Geometry check sheet. Reference: the model listing, model coordinates, mm. Face numbers are marked on the shaded views. Give positions to 0.01 mm unless a question says otherwise; leave off trailing zeros. Order: outer loops, then holes, each group sorted by start corner. A loop starts at its lowest first (then second) coordinate and runs counter-clockwise, first axis right, second up. Notation, with made-up numbers: (16, 47) - (70, 47) arc R23 ccw to (70, 73) - close; hole circle Ø2 at (-10.75, 27.5). An arc over 180 degrees is marked (long way). Put each result on its own line as item: value. Start each with the question number.
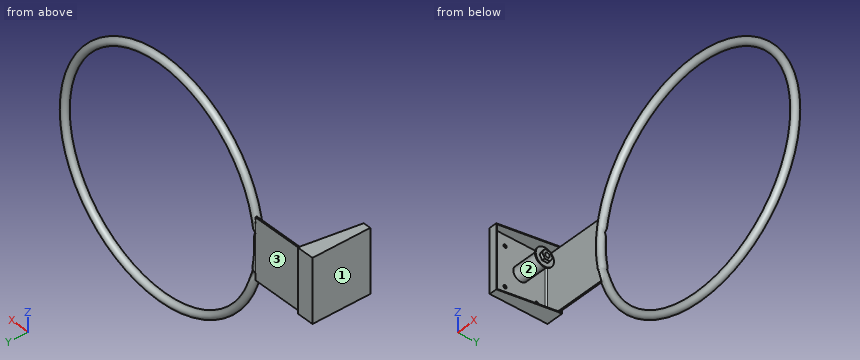
Autodesk Inventor part; units mm, degrees
ref_plane "YZ Plane" through (0, 0, 0) normal (1, 0, 0) x (0, 1, 0)
ref_plane "XZ Plane" through (0, 0, 0) normal (0, 1, 0) x (-1, 0, 0)
ref_plane "XY Plane" through (0, 0, 0) normal (0, 0, 1) x (1, 0, 0)
sketch "Sketch1" plane through (0, 0, 0) normal (0, 0, 1) x (1, 0, 0)
  circle A0 centre (0, 0) radius 7.9375
  line L0 (236.5375, 47.7842) -> (236.5375, -114.9552)
  dimension "d0" = 228.6
  dimension "d1" = 15.875
revolve "Revolution1" add sketch "Sketch1" angle 360 about axis through (236.5375, 47.7842, 0) along (0, -1, 0)
sketch "Sketch2" plane through (0, 0, 0) normal (0, 0, 1) x (1, 0, 0)
  line L0 (0, 4.7625) -> (-134.9375, 4.7625)
  line L1 (-138.1125, 1.5875) -> (-138.1125, -106.3625)
  line L2 (-138.1125, -106.3625) -> (-141.2875, -106.3625)
  line L3 (-141.2875, -106.3625) -> (-141.2875, 1.5875)
  line L4 (-134.9375, 7.9375) -> (0, 7.9375)
  line L5 (0, 7.9375) -> (0, 4.7625)
  arc A0 (-134.9375, 4.7625) -> (-138.1125, 1.5875) centre (-134.9375, 1.5875) ccw
  arc A1 (-134.9375, 7.9375) -> (-141.2875, 1.5875) centre (-134.9375, 1.5875) ccw
  point P0 (0, 0)
  point P1 (-138.1125, 4.7625)
  dimension "d5" = 0
  dimension "d6" = 7.9375
  dimension "d7" = 3.175
  dimension "d8" = 3.175
  dimension "d9" = 6.35
  dimension "d27" = 114.3
  dimension "d28" = 141.2875
extrude "Extrusion1" add sketch "Sketch2" along normal mid plane 125.4125
sketch "Sketch3" plane through (-141.2875, -106.3625, 62.7062) normal (-1, 0, 0) x (0, 0, 1)
  line L0 (0, 0) -> (0, 107.95)
  line L1 (0, 107.95) -> (-125.4125, 107.95)
  line L2 (-125.4125, 107.95) -> (-125.4125, 0)
  line L3 (0, 0) -> (-125.4125, 0)
  line L4 (0, 114.3) -> (-125.4125, 114.3)
  line L5 (-125.4125, 107.95) -> (-125.4125, 114.3)
  line L6 (0, 114.3) -> (0, 107.95)
  arc A0 (-103.9113, 100.9746) -> (-110.4012, 84.7629) centre (-107.1562, 92.8687) ccw
  arc A1 (-102.47, 81.5879) -> (-95.9802, 97.7996) centre (-99.2251, 89.6937) ccw
  arc A2 (-29.4323, 97.7996) -> (-22.9425, 81.5879) centre (-26.1874, 89.6937) ccw
  arc A3 (-15.0113, 84.7629) -> (-21.5012, 100.9746) centre (-18.2562, 92.8687) ccw
  arc A4 (-110.4012, 31.1246) -> (-103.9113, 14.9129) centre (-107.1562, 23.0187) ccw
  arc A5 (-95.9802, 18.0879) -> (-102.47, 34.2996) centre (-99.2251, 26.1937) ccw
  arc A6 (-22.9425, 34.2996) -> (-29.4323, 18.0879) centre (-26.1874, 26.1937) ccw
  arc A7 (-21.5012, 14.9129) -> (-15.0113, 31.1246) centre (-18.2562, 23.0187) ccw
  line L7 (-110.4012, 84.7629) -> (-102.47, 81.5879)
  line L8 (-103.9113, 100.9746) -> (-95.9802, 97.7996)
  line L9 (-21.5012, 100.9746) -> (-29.4323, 97.7996)
  line L10 (-15.0113, 84.7629) -> (-22.9425, 81.5879)
  line L11 (-22.9425, 34.2996) -> (-15.0113, 31.1246)
  line L12 (-21.5012, 14.9129) -> (-29.4323, 18.0879)
  line L13 (-103.9113, 14.9129) -> (-95.9802, 18.0879)
  line L14 (-102.47, 34.2996) -> (-110.4012, 31.1246)
  line L15 (-107.1562, 23.0187) -> (-107.1562, 92.8687)
  line L16 (-99.2251, 26.1937) -> (-99.2251, 89.6937)
  line L17 (-26.1874, 26.1937) -> (-26.1874, 89.6937)
  line L18 (-18.2562, 23.0187) -> (-18.2562, 92.8687)
  line L19 (-99.2251, 89.6937) -> (-26.1874, 89.6937)
  line L20 (-107.1562, 92.8687) -> (-18.2562, 92.8687)
  line L21 (-99.2251, 26.1937) -> (-26.1874, 26.1937)
  line L22 (-107.1562, 23.0187) -> (-18.2562, 23.0187)
  dimension "d29" = 106.3625
  dimension "d30" = 55.5752
  dimension "d31" = 87.3125
  dimension "d32" = 46.0375
  dimension "d33" = 17.4625
  dimension "d34" = 9.525
  dimension "d35" = 12.7
  dimension "d36" = 9.525
  dimension "d37" = 33.3375
  dimension "d38" = 79.375
  dimension "d39" = 34.9186
hole "Hole1" at (-138.1125, -15.0812, 40.4812) direction (-1, 0, 0) diameter 6.731 end through all
pattern_linear "Rectangular Pattern1" count 2 spacing 80.9625 along (0, 0, -1) count 2 spacing 66.675 along (0, -1, 0) of "Hole1"
hole "Hole2" at (-141.2875, -49.2125, 0.7937) direction (1, 0, 0) diameter 12.7 depth 25.4 tip angle 118
sketch "Sketch4" plane through (-141.2875, -106.3625, 62.7062) normal (-1, 0, 0) x (0, 0, 1)
  line L0 (0, 0) -> (0, 107.95)
  line L1 (-125.4125, 107.95) -> (-125.4125, 0)
  line L2 (0, 0) -> (-125.4125, 0)
  line L3 (-128.5875, -3.175) -> (3.175, -3.175)
  line L4 (3.175, -3.175) -> (3.175, 117.475)
  line L5 (3.175, 117.475) -> (-128.5875, 117.475)
  line L6 (-128.5875, 117.475) -> (-128.5875, -3.175)
  line L7 (0, 114.3) -> (-125.4125, 114.3)
  line L8 (-127, 115.8875) -> (1.5875, 115.8875)
  line L9 (1.5875, 115.8875) -> (1.5875, -1.5875)
  line L10 (1.5875, -1.5875) -> (-127, -1.5875)
  line L11 (-127, -1.5875) -> (-127, 115.8875)
  point P0 (-62.7062, 106.3625)
  dimension "d49" = 3.175
  dimension "d50" = 3.175
  dimension "d51" = 3.175
  dimension "d52" = 3.175
  dimension "d53" = 1.5875
extrude "Extrusion2" add sketch "Sketch4" along normal blind 1.5875 contours L6 L5 L4 L3 | L8 L9 L10 L11
extrude "Extrusion3" add sketch "Sketch4" against normal blind 33.3375
sketch "Sketch8" plane through (-142.875, -109.5375, 65.8813) normal (0, 0, 1) x (1, 0, 0)
  line L0 (0, 120.65) -> (0, 0)
  line L1 (34.925, 0) -> (0, 0)
  line L2 (34.925, 0) -> (34.925, 120.65)
  line L3 (34.925, 120.65) -> (0, 120.65)
  line L4 (34.925, 114.3) -> (15.875, 0)
  line L5 (34.925, 0) -> (34.925, 114.3)
  line L6 (15.875, 0) -> (34.925, 0)
  point P0 (142.875, 109.5375)
  dimension "d67" = 6.35
  dimension "d68" = 15.875
extrude "Extrusion7" cut sketch "Sketch8" against normal through all contours L4 L2 L1
sketch "Sketch5" plane through (-141.2875, -49.2125, 0.7937) normal (1, 0, 0) x (0, 0, -1)
  circle A0 centre (0, 0) radius 6.35
  circle A1 centre (0, 0) radius 4.7625
  point P0 (0.7937, 49.2125)
  dimension "d58" = 9.525
extrude "Extrusion4" add sketch "Sketch5" along normal blind 60.325 contours A1
sketch "Sketch6" plane through (-80.9625, -49.2125, 0.7937) normal (1, 0, 0) x (0, 0, -1)
  circle A0 centre (0, 0) radius 4.7625
  circle A1 centre (0, 0) radius 19.05
  point P0 (0.7937, 49.2125)
  dimension "d61" = 38.1
extrude "Extrusion5" add sketch "Sketch6" along normal blind 1.905
sketch "Sketch7" plane through (-79.0575, -49.2125, 0.7937) normal (1, 0, 0) x (0, 0, -1)
  circle A0 centre (0, 0) radius 4.7625
  circle A1 centre (0, 0) radius 19.05
  line L0 (0, 10.9985) -> (9.525, 5.4993)
  line L1 (9.525, 5.4993) -> (9.525, -5.4993)
  line L2 (9.525, -5.4993) -> (0, -10.9985)
  line L3 (0, -10.9985) -> (-9.525, -5.4993)
  line L4 (-9.525, -5.4993) -> (-9.525, 5.4993)
  line L5 (-9.525, 5.4993) -> (0, 10.9985)
  point P0 (0.7937, 49.2125)
  dimension "d64" = 19.05
extrude "Extrusion6" add sketch "Sketch7" along normal blind 6.35 contours L0 L1 L2 L3 L4 L5
sketch "Sketch9" plane through (-138.1125, -106.3625, 62.7062) normal (1, 0, 0) x (0, 0, -1)
  circle A0 centre (61.9125, 57.15) radius 6.35
  circle A1 centre (61.9125, 57.15) radius 15.0812
  circle A2 centre (61.9125, 57.15) radius 8.7313
  point P0 (62.7062, 106.3625)
  dimension "d71" = 30.1625
  dimension "d72" = 17.4625
extrude "Extrusion8" add sketch "Sketch9" along normal blind 57.15 contours A1
equation "\"d50\" = d49"
equation "\"d51\" = d49"
equation "\"d52\" = d49"
properties part number "GE-12013"
Item 1: Cross-section at A-A (x = -98). Enter the section's corners in (y, z) (1 decimal).
Item 2: Thickness scan on line 1 along X through (y, z) = (-54, 61.5) (1 decimal); line 2 along Z through (x, y) = (336, 0); line 3 along Y through (x, z) = (83, -176). Record the ranges inside material, lowest first.
Item 3: Cross-section at C-C (x = -21.5). Enter the section's corners in (y, z), and give its area (3 significant figures).
Item 4: Release check for a two-part mould opening along X. For the marked faces 1, 2 and 3 record: +X half, -X half, draft (parallel to the pull), parting line (faces both ways), or undercut.
Item 5: Gauge pin test, flat ends, axial feed: pin 1 Ø1.5 at (y, z) = (-37.5, 30) entering from +X; pin 2 Ø8 at (x, z) = (-79, 9.5) entering from -Y; pin 3 Ø2 at (y, z) = (-15, -41.5) entering from +X. Record the tip position at first contact, or that the pin passes through.
Item 6: Cross-section at B-B (y = -99). Enter the section's corners in (x, z) (1 decimal), and give its area (3 significant figures).
Recorded:
1. outline: circle Ø30.2 at (-49.2, 0.8); circle Ø9.5 at (-49.2, 0.8); (4.8, -62.7) - (7.9, -62.7) - (7.9, 62.7) - (4.8, 62.7) - close; hole circle Ø17.5 at (-49.2, 0.8)
2. line 1: x = -142.9 to -138.1
2. line 2: z = -223.33 to -205.83, 205.83 to 223.33
2. line 3: y = -7.36 to 7.36
3. outline: (4.76, -62.71) - (7.94, -62.71) - (7.94, 62.71) - (4.76, 62.71) - close
3. area: 398 mm^2
4. face 1: -X half
4. face 2: undercut
4. face 3: draft
5. pin 1: stops at x = -138.11
5. pin 2: stops at y = -67.67
5. pin 3: stops at x = -141.29
6. outline: (-142.9, -65.9) - (-125.2, -65.9) - (-125.2, -64.3) - (-141.3, -64.3) - (-141.3, -62.7) - (-138.1, -62.7) - (-138.1, 62.7) - (-141.3, 62.7) - (-141.3, 64.3) - (-125.2, 64.3) - (-125.2, 65.9) - (-142.9, 65.9) - close
6. area: 658 mm^2
